```python
from build123d import *

# Parameters (mm, degrees)
F0_W     = 190.5
F0_H     = 139.7
F1_DEPTH = 101.6
F2_R     = 25.4
F3_DEPTH = 152.401


# Not quite as in the source:
# - ends of sketch curves that miss each other by under 0.0002 mm in the source are joined


with BuildPart() as f1:
    # F0 (on Front) → F1 (new body)
    with BuildSketch(Plane.XZ):
        with BuildLine():
            Line((-95.25, -76.2), (95.25, -76.2))
            ThreePointArc((95.25, -76.2), (99.7401280605, -74.3401280605), (101.6, -69.85))
            Line((101.6, -69.85), (101.6, 69.85))
            ThreePointArc((101.6, 69.85), (99.7401280605, 74.3401280605), (95.25, 76.2))
            Line((95.25, 76.2), (-95.25, 76.2))
            ThreePointArc((-95.25, 76.2), (-99.7401280605, 74.3401280605), (-101.6, 69.85))
            Line((-101.6, 69.85), (-101.6, -69.85))
            ThreePointArc((-101.6, -69.85), (-99.7401280605, -74.3401280605), (-95.25, -76.2))
        make_face()
        Rectangle(F0_W, F0_H, mode=Mode.SUBTRACT)
    extrude(amount=F1_DEPTH)

    # F2 (on face) → F3 (cut, through all)
    with BuildSketch(Plane.XY.offset(76.2)):
        with Locations((0, -50.8)):
            Circle(F2_R)
    extrude(amount=-F3_DEPTH, mode=Mode.SUBTRACT)


solid = f1.part
```
Geometry check sheet. Reference: the model listing, model coordinates, mm. A direction names the side the tool comes from. Coordinates: 2 decimals unless noted, no trailing zeros. Order: outer loops, then holes, each group sorted by start corner. A loop starts at its lowest first (then second) coordinate and runs counter-clockwise, first axis right, second up. Notation, with made-up numbers: (44, -12) - (98, -12) arc R3 ccw to (98, -8) - close; hole circle Ø11 at (50.25, 46.25). An arc over 180 degrees is marked (long way). Answer in a Markdown table with one row per item. Add a question column.
1. Access from +Z, -Z, +X, -X, +Y, -Y to the whole of each face (thin tool, end or side, straight path). Record for faces 5 (the face through (-23, -39, -69.85)), 6 (the face through (99.69, -50.09, -74.39)).
2. Material ranges on L1, parallel to Y at x = 0, z = 74.25; L2, parallel to X at y = -34, z = -42; L3, parallel to Z at x = 66.5, y = -29.5, recorded low to high. Write a range as [from, to].
3. Section check C-C (x = 0). Enter the section's corners in (y, z), plus the area to 3 significant figures.
4. Section check A-A (z = -54). Enter the section's corners in (x, y), plus the area to 3 significant figures.
5. Section check D-D (y = -11.5). Enter the section's corners in (x, z).
6. Section check B-B (x = 36.5). Enter the section's corners in (y, z).
7. Draft check along X on faces 1 (the face through (95.25, -50, -1)), 2 (the face through (99.79, -50.09, 74.29)), 3 (the face through (-99.69, -50.09, 74.39)), 4 (the face through (-8, -101.6, -73)). Enter one of: +X half, -X half, draft (parallel to the pull), parting line (faces both ways), or undercut.
Data:
| question | item | result |
|---|---|---|
| 1 | face 5 | +Y, -Y |
| 1 | face 6 | -Z, +X, +Y, -Y |
| 2 | L1 | y = [-101.6, -76.2], [-25.4, 0] |
| 2 | L2 | x = [-101.6, -95.25], [95.25, 101.6] |
| 2 | L3 | z = [-76.2, -69.85], [69.85, 76.2] |
| 3 | outline | (-101.6, -76.2) - (-76.2, -76.2) - (-76.2, -69.85) - (-101.6, -69.85) - close; (-101.6, 69.85) - (-76.2, 69.85) - (-76.2, 76.2) - (-101.6, 76.2) - close; (-25.4, -76.2) - (0, -76.2) - (0, -69.85) - (-25.4, -69.85) - close; (-25.4, 69.85) - (0, 69.85) - (0, 76.2) - (-25.4, 76.2) - close |
| 3 | area | 645 mm² |
| 4 | outline | (-101.6, -101.6) - (-95.25, -101.6) - (-95.25, 0) - (-101.6, 0) - close; (95.25, -101.6) - (101.6, -101.6) - (101.6, 0) - (95.25, 0) - close |
| 4 | area | 1,290 mm² |
| 5 | outline | (-101.6, -69.85) arc R6.35 ccw to (-95.25, -76.2) - (95.25, -76.2) arc R6.35 ccw to (101.6, -69.85) - (101.6, 69.85) arc R6.35 ccw to (95.25, 76.2) - (-95.25, 76.2) arc R6.35 ccw to (-101.6, 69.85) - close; hole (-95.25, -69.85) - (95.25, -69.85) - (95.25, 69.85) - (-95.25, 69.85) - close |
| 6 | outline | (-101.6, -76.2) - (0, -76.2) - (0, -69.85) - (-101.6, -69.85) - close; (-101.6, 69.85) - (0, 69.85) - (0, 76.2) - (-101.6, 76.2) - close |
| 7 | face 1 | undercut |
| 7 | face 2 | +X half |
| 7 | face 3 | -X half |
| 7 | face 4 | draft |
